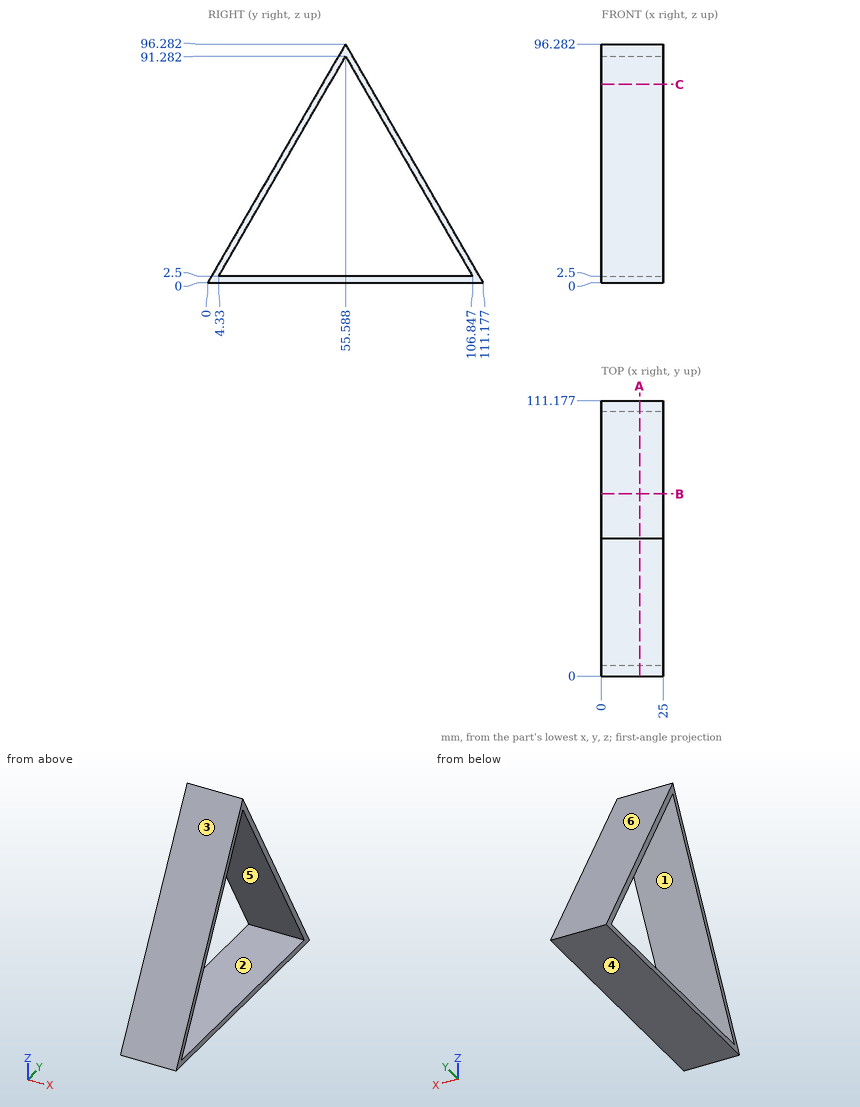
Print and shaded views of the part. All mm, measured from the part's lowest x, y and z. A direction names the side the tool comes from. Round coordinates to 2 decimals unless told otherwise and drop trailing zeros. Write each loop counter-clockwise with the first axis right and the second up, starting at its lowest first coordinate (ties: lowest second). Pieces come first, ordered by that corner, then holes. Notation, with made-up numbers: (49.25, 70.5) -> (62.25, 70.5) arc R22 ccw to (62.25, 105.5) -> close; hole circle Ø4 at (27.25, 81). An arc over 180 degrees is marked (long way). Return JSON: item names as keys, results as strings. Group by question number.
Q1. Saw through at C-C on z = 80. Write the cut outline in (x, y) (1 decimal), plus the area to 3 significant figures.
Q2. Pin check, flat tips, straight feed: pin 1 (12 mm diameter, centred on y = 64, z = 77.5, fed in from -X); pin 2 (6 mm diameter, centred on x = 11, y = 39.5, fed in from +Z) (1 decimal); pin 3 (10 mm diameter, centred on x = 22.5, z = 77.5, fed in from -Y); pin 4 (5 mm diameter, centred on x = 20, z = 71, fed in from -Y). Stop position of each tip, or through.
Q3. Saw through at B-B on y = 73.5. Write the cut outline in (x, z).
Q4. Probe L1, parallel to Y at x = 22.5, z = 49 (1 decimal); L2, parallel to Y at x = 13, z = 58.5 (1 decimal); L3, parallel to Z at x = 3.25, y = 71.5 (1 decimal). List the from-to ranges inside material, lowest first. Write a range as [from, to].
Q5. Saw through at A-A on x = 15.5. Write the cut outline in (y, z).
Q6. Mould opens along Y. For the marked faces 1, 2, 3 and 4 say: pulls with the +Y half, pulls with the -Y half, needs draft (parallel to the pull), parting line crosses it, or undercut.
Q7. Which spindle directions (+Z, -Z, +X, -X, +Y, -Y) get a long thin tool onto all of the face, cutting with end or side? Do the marked faces 5 and 6. Say none if no direction does.
Answer:
{
 "1": {"outline": "(0, 46.2) -> (25, 46.2) -> (25, 49.1) -> (0, 49.1) -> close; (0, 62.1) -> (25, 62.1) -> (25, 65) -> (0, 65) -> close", "area": "144 mm2"},
 "2": {"pin 1": "x = 0", "pin 2": "z = 73.6", "pin 3": "y = 41.86", "pin 4": "y = 39.55"},
 "3": {"outline": "(0, 0) -> (25, 0) -> (25, 2.5) -> (0, 2.5) -> close; (0, 60.26) -> (25, 60.26) -> (25, 65.26) -> (0, 65.26) -> close"},
 "4": {"L1": "[28.3, 31.2], [80, 82.9]", "L2": "[33.8, 36.7], [74.5, 77.4]", "L3": "[0, 2.5], [63.7, 68.7]"},
 "5": {"outline": "(0, 0) -> (111.18, 0) -> (55.59, 96.28) -> close; hole (4.33, 2.5) -> (106.85, 2.5) -> (55.59, 91.28) -> close"},
 "6": {"face 1": "undercut", "face 2": "undercut", "face 3": "pulls with the -Y half", "face 4": "needs draft"},
 "7": {"face 5": "+X, -X", "face 6": "+Z, +X, -X, +Y"}
}
